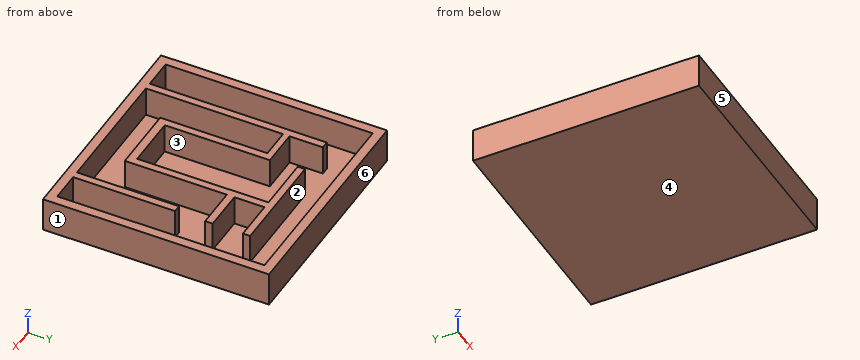
from build123d import *

# Parameters (mm, degrees)
F0_W      = 38.1
F0_H      = 38.1
F1_DEPTH  = 0.79375
F2_W      = 38.1
F2_H      = 38.1
F2_W_2    = 34.925
F2_H_2    = 34.925
F3_DEPTH  = 5.08
F4_W      = 1.27
F4_H      = 29.845
F5_DEPTH  = 5.08
F6_R      = 1.27
F7_DEPTH  = 0.396875
F9_DEPTH  = 5.08
F8_W      = 1.27
F8_H      = 17.1959060269
F10_DEPTH = 5.08
F8_R      = 1.27
F11_DEPTH = 0.396875
F8_W_2    = 6.985
F8_H_2    = 1.27
F12_DEPTH = 5.08


# Not quite as in the source:
# - a feature names something its author has since deleted; it is built from what else it names


with BuildPart() as f1:
    # F0 (on Top) → F1 (new body)
    with BuildSketch(Plane.XY):
        with Locations((-16.4964904517, -15.5271535208)):
            Rectangle(F0_W, F0_H)
    extrude(amount=F1_DEPTH)

    # F2 (on face) → F3 (join)
    with BuildSketch(Plane.XY.offset(0.79375)):
        with Locations((-16.4964904517, -15.5271535208)):
            Rectangle(F2_W, F2_H)
        with Locations((-16.4964904517, -15.5271535208)):
            Rectangle(F2_W_2, F2_H_2, mode=Mode.SUBTRACT)
    extrude(amount=F3_DEPTH)

    # F4 (on face) → F5 (join)
    with BuildSketch(Plane.XY.offset(0.79375)):
        with Locations((-28.2439904517, -18.0671535208)):
            Rectangle(F4_W, F4_H)
    extrude(amount=F5_DEPTH)

    # F6 (on face) → F7 (cut)
    with BuildSketch(Plane.XY.offset(0.79375)):
        with Locations((-31.4189904517, -30.6663066149)):
            Circle(F6_R)
    extrude(amount=-F7_DEPTH, mode=Mode.SUBTRACT)

    # F8 (on face) → F9 (join)
    with BuildSketch(Plane.XY.offset(0.79375)):
        Polygon((-4.1139904517, -3.1446535208), (-21.8377289305, -3.1446535208), (-21.8377289305, -4.3637474939), (-12.3689904517, -4.3637474939), (-12.3689904517, -26.4913998544), (-21.2589904517, -26.4913998544), (-21.2589904517, -8.7657477707), (-22.5289904517, -8.7657477707), (-27.6089904517, -8.7657477707), (-27.6089904517, -9.8523776978), (-22.5289904517, -9.8523776978), (-22.5289904517, -27.9096535208), (-11.0989904517, -27.9096535208), (-11.0989904517, -10.7137474939), (-11.0989904517, -9.4437474939), (-11.0989904517, -4.3637474939), (-4.1139904517, -4.3637474939), align=None)
    extrude(amount=F9_DEPTH)

    # F8 (on face) → F10 (join)
    with BuildSketch(Plane.XY.offset(0.79375)):
        with Locations((-4.7489904517, -24.3917005073)):
            Rectangle(F8_W, F8_H)
    extrude(amount=F10_DEPTH)

    # F8 (on face) → F11 (cut)
    with BuildSketch(Plane.XY.offset(0.79375)):
        with Locations((-25.0689904517, -13.1018003449)):
            Circle(F8_R)
    extrude(amount=-F11_DEPTH, mode=Mode.SUBTRACT)

    # F8 (on face) → F12 (join)
    with BuildSketch(Plane.XY.offset(0.79375)):
        with Locations((-7.6064904517, -10.0787474939)):
            Rectangle(F8_W_2, F8_H_2)
    extrude(amount=F12_DEPTH)


solid = f1.part
Input: part model. Units: mm. Frame: model coordinates. Face numbers are marked on the shaded views. A direction names the side the tool comes from. Give positions to 0.01 mm unless a question says otherwise; leave off trailing zeros. Loops run counter-clockwise (first coordinate to the right, second up) from the corner with the lowest first, then second, coordinate; pieces in that order, holes last. Notation, with made-up numbers: M 78.25,65 L 93.25,65 A20 cw 93.25,90 Z; hole C 74.25,38 d10. An arc over 180 degrees is marked long. Use one line per item in the form item = value.
1. Pull-direction query (Y, two-part tool) for the marked faces 3, 4, 5 and 6; classes: released by +Y, released by -Y, zero draft, split by the parting line, or undercut.
Numbers:
face_3 = undercut
face_4 = zero draft
face_5 = released by -Y
face_6 = released by +Y
2. Section query D-D, the plane y = 0. Return the cut outline in (x, z).
Numbers:
outline = M -35.55,0 L 2.55,0 L 2.55,5.87 L 0.97,5.87 L 0.97,0.79 L -33.96,0.79 L -33.96,5.87 L -35.55,5.87 Z
3. Reachability of the marked faces 1 and 2 from +Z, -Z, +X, -X, +Y, -Y: full face, straight path, thin tool, end or side. Return the list, or none.
Numbers:
face_1 = +Z, -Z, +X, +Y, -Y
face_2 = +Z
4. First-contact query: pin 1 (1.5 mm diameter, centred on x = -27, y = -19, fed in from +Z); pin 2 (1 mm diameter, centred on x = -9.5, y = -19, fed in from +Z); pin 3 (2 mm diameter, centred on x = -31.42, y = -30.67, fed in from +Z). Flat tips, straight axial feed; report the tip coordinate or a pass-through.
Numbers:
pin_1 = 5.87
pin_2 = 0.79
pin_3 = 0.4
5. Line query: L1, parallel to Y at x = -13.5, z = 5.2; L2, parallel to X at y = -4, z = 4.6; L3, parallel to Y at x = -9.5, z = 4.75. Output: solid intervals per line, ascending.
Numbers:
L1 = -34.58 to -32.99, -27.91 to -26.49, -4.36 to -3.14, 1.94 to 3.52
L2 = -35.55 to -33.96, -28.88 to -27.61, -21.84 to -4.11, 0.97 to 2.55
L3 = -34.58 to -32.99, -10.71 to -9.44, -4.36 to -3.14, 1.94 to 3.52
6. Section query C-C, the plane y = -17.5. Return the cut outline in (x, z).
Numbers:
outline = M -35.55,0 L 2.55,0 L 2.55,5.87 L 0.97,5.87 L 0.97,0.79 L -4.11,0.79 L -4.11,5.87 L -5.38,5.87 L -5.38,0.79 L -11.1,0.79 L -11.1,5.87 L -12.37,5.87 L -12.37,0.79 L -21.26,0.79 L -21.26,5.87 L -22.53,5.87 L -22.53,0.79 L -27.61,0.79 L -27.61,5.87 L -28.88,5.87 L -28.88,0.79 L -33.96,0.79 L -33.96,5.87 L -35.55,5.87 Z
7. Section query B-B, the plane x = -1. Return the cut outline in (y, z).
Numbers:
outline = M -34.58,0 L 3.52,0 L 3.52,5.87 L 1.94,5.87 L 1.94,0.79 L -32.99,0.79 L -32.99,5.87 L -34.58,5.87 Z
